```python
from build123d import *

# Parameters (mm, degrees)
F0_R     = 49.53
F0_R_2   = 44.45
F1_DEPTH = 25.4
F3_DEPTH = 17.5
F4_R     = 2


with BuildPart() as f1:
    # F0 (on Top) → F1 (new body)
    with BuildSketch(Plane.XY):
        Circle(F0_R)
        Circle(F0_R_2, mode=Mode.SUBTRACT)
    extrude(amount=F1_DEPTH)

    # F2 (on Right) → F3 (join, symmetric)
    with BuildSketch(Plane.YZ):
        Polygon((66.002712847, 25.4), (45.682712847, 25.4), (45.682712847, 16.2404105067), (60.96, 16.2404105067), (60.96, -37.6108922064), (66.002712847, -38.1), align=None)
    extrude(amount=F3_DEPTH, both=True)

    # F4
    f4_edges = [f1.edges().sort_by_distance(p)[0] for p in [
        (0, 60.96, 16.240411),
        (0, 49.53, 16.240411),
        (17.5, 46.335417, 20.820205),
        (-17.5, 46.335417, 20.820205),
        (0, 66.002713, 25.4),
        (-44.45, 0, 25.4),
        (-49.53, 0, 0),
        (49.53, 0, 12.7),
        (-28.164214, -40.743072, 25.4),
        (40.743072, 28.164214, 25.4),
        (44.45, 0, 12.7),
        (-44.45, 0, 0),
        (-17.5, 66.002713, -6.35),
        (17.5, 66.002713, -6.35),
        (0, 66.002713, -38.1),
        (17.5, 56.169065, 25.4),
        (-17.5, 56.169065, 25.4),
    ]]
    fillet(f4_edges, radius=F4_R)


solid = f1.part
```
Geometry check sheet. Reference: the model listing, model coordinates, mm. A direction names the side the tool comes from. Round coordinates to 2 decimals unless told otherwise and drop trailing zeros. Loops run counter-clockwise (first coordinate to the right, second up) from the corner with the lowest first, then second, coordinate; pieces in that order, holes last. Notation, with made-up numbers: (13.25, 89.5) - (52.25, 89.5) arc R29 ccw to (52.25, 119.5) - close; hole circle Ø5 at (12, 89.25). An arc over 180 degrees is marked (long way). Write each question's results on one line, items separated by ' | '. Start each with the question number.
Q1. Cross-section at C-C on y = 0. Enter the section's corners in (x, z), and give its area (3 significant figures).
Q2. Access from +Z, -Z, +X, -X, +Y, -Y to the whole of each face (thin tool, end or side, straight path). Record for faces 1 (the flat face through (17.5, 61.2, -0.3)), 2 (the flat face through (10, -46, 0)), 3 (the cylindrical face through (42.397, 13.352, 12.55)).
Q3. Cross-section at A-A on z = 6.5. Enter the section's corners in (x, y).
Q4. Release check for a two-part mould opening along Y. For faces 4 (the flat face through (0, 66.003, -7)), 5 (the flat face through (-17.5, 61.2, -0.3)), 6 (the flat face through (0, 60.96, -11)), 7 (the flat face through (0, 55, 16.24)) record: +Y half, -Y half, draft (parallel to the pull), parting line (faces both ways), or undercut.
Q5. Cross-section at D-D on z = 18. Enter the section's corners in (x, y), and give its area (3 significant figures).
Q6. Gauge pin test, flat ends, axial feed: P1, Ø11.5, axis at x = 5.5, y = 56, coming from the -Z side; P2, Ø1, axis at y = -28, z = -1.5, coming from the +X side; P3, Ø2, axis at y = -20.5, z = 4.5, coming from the -X side; P4, Ø3, axis at y = 23, z = 13, coming from the -X side. Record the tip position at first contact, or that the pin passes through.
Q7. Thickness scan on line 1 (Y direction, x = 0, z = 8.5); line 2 (Y direction, x = 13, z = 10); line 3 (Z direction, x = -10.5, y = 60.5). Record the ranges inside material, lowest first. Write a range as [from, to].
Q8. Cross-section at B-B on x = 0. Enter the section's corners in (y, z).
Answers below:
1) outline: (-49.53, 2) arc R2 ccw to (-47.53, 0) - (-46.45, 0) arc R2 ccw to (-44.45, 2) - (-44.45, 23.4) arc R2 ccw to (-46.45, 25.4) - (-47.53, 25.4) arc R2 ccw to (-49.53, 23.4) - close; (44.45, 2) arc R2 ccw to (46.45, 0) - (47.53, 0) arc R2 ccw to (49.53, 2) - (49.53, 23.4) arc R2 ccw to (47.53, 25.4) - (46.45, 25.4) arc R2 ccw to (44.45, 23.4) - close | area: 251 mm²
2) face 1: +Z, -Z, +X, +Y | face 2: -Z, +X, -X, -Y | face 3: +Z, -Z
3) outline: circle Ø99.06 at (0, 0); (-17.5, 60.96) - (17.5, 60.96) - (17.5, 64) arc R2 ccw to (15.5, 66) - (-15.5, 66) arc R2 ccw to (-17.5, 64) - close; hole circle Ø88.9 at (0, 0)
4) face 4: +Y half | face 5: draft | face 6: undercut | face 7: undercut
5) outline: (-18.74, 45.85) arc R49.53 ccw (long way) to (18.74, 45.85) arc R2 cw to (17.5, 47.7) - (17.5, 64) arc R2 ccw to (15.5, 66) - (-15.5, 66) arc R2 ccw to (-17.5, 64) - (-17.5, 47.7) arc R2 cw to start; hole circle Ø88.9 at (0, 0) | area: 2,110 mm²
6) P1: stops at z = -37.69 | P2: passes through | P3: stops at x = -45.53 | P4: stops at x = -44.62
7) line 1: y = [-49.53, -44.45], [44.45, 49.53], [60.96, 66] | line 2: y = [-47.79, -42.51], [42.51, 47.79], [60.96, 66] | line 3: z = [15.52, 25.4]
8) outline: (-49.53, 2) arc R2 ccw to (-47.53, 0) - (-46.45, 0) arc R2 ccw to (-44.45, 2) - (-44.45, 23.4) arc R2 ccw to (-46.45, 25.4) - (-47.53, 25.4) arc R2 ccw to (-49.53, 23.4) - close; (44.45, 2) arc R2 ccw to (46.45, 0) - (47.53, 0) arc R2 ccw to (49.53, 2) - (49.53, 14.24) arc R2 cw to (51.53, 16.24) - (58.96, 16.24) arc R2 cw to (60.96, 14.24) - (60.96, -37.61) - (63.81, -37.89) arc R2 ccw to (66, -35.9) - (66, 23.4) arc R2 ccw to (64, 25.4) - (46.45, 25.4) arc R2 ccw to (44.45, 23.4) - close
